Here's how the part is built. I have some questions about the finished solid (model axes, mm). A direction names the side the tool comes from. Round coordinates to 2 decimals unless told otherwise and drop trailing zeros. Write each loop counter-clockwise with the first axis right and the second up, starting at its lowest first coordinate (ties: lowest second). Pieces come first, ordered by that corner, then holes. Notation, with made-up numbers: M 23.5,78 L 72.5,78 A22 ccw 72.5,97 Z; hole C 25,58.5 d1. An arc over 180 degrees is marked long. Use a Markdown table: item, result. Add a question column.
```python
from build123d import *

# Parameters (mm, degrees)
F0_W      = 25
F0_H      = 27.7
F0_H_2    = 25
F0_W_2    = 27.7
F1_DEPTH  = 2
F0_W_3    = 1.8
F2_DEPTH  = 130
F0_H_3    = 1.8
F3_DEPTH  = 4
F4_W      = 25
F4_H      = 2
F5_DEPTH  = 80.4
F7_W      = 25
F7_H      = 2
F8_DEPTH  = 25
F6_W      = 25
F6_H      = 2
F9_DEPTH  = 25
F12_DEPTH = 25
F13_R     = 5


with BuildPart() as f1:
    # F0 (on Top) → F1 (new body)
    with BuildSketch(Plane.XY):
        with Locations((0, 26.35)):
            Rectangle(F0_W, F0_H)
        Rectangle(F0_W, F0_H_2)
        with Locations((26.35, 0)):
            Rectangle(F0_W_2, F0_H_2)
        with Locations((0, -26.35)):
            Rectangle(F0_W, F0_H)
        with Locations((-26.35, 0)):
            Rectangle(F0_W_2, F0_H_2)
    extrude(amount=F1_DEPTH)

    # F0 (on Top) → F2 (join)
    with BuildSketch(Plane.XY):
        with Locations((-41.1, 0)):
            Rectangle(F0_W_3, F0_H_2)
        with Locations((41.1, 0)):
            Rectangle(F0_W_3, F0_H_2)
    extrude(amount=F2_DEPTH)

    # F0 (on Top) → F3 (join)
    with BuildSketch(Plane.XY):
        with Locations((0, 41.1)):
            Rectangle(F0_W, F0_H_3)
        with Locations((0, -41.1)):
            Rectangle(F0_W, F0_H_3)
    extrude(amount=F3_DEPTH)

    # F4 (on face) → F5 (join)
    with BuildSketch(Plane(origin=(40.2, 0, 0), x_dir=(0, -1, 0), z_dir=(-1, 0, 0))):
        with Locations((0, 129)):
            Rectangle(F4_W, F4_H)
    extrude(amount=F5_DEPTH)

    # F7 (on face) → F8 (join)
    with BuildSketch(Plane.YZ.offset(42)):
        with Locations((0, 129)):
            Rectangle(F7_W, F7_H)
    extrude(amount=F8_DEPTH)

    # F6 (on face) → F9 (join)
    with BuildSketch(Plane(origin=(-42, 0, 0), x_dir=(0, -1, 0), z_dir=(-1, 0, 0))):
        with Locations((0, 129)):
            Rectangle(F6_W, F6_H)
    extrude(amount=F9_DEPTH)

    # F11 (on face) + F10 (on face) → F12 (cut)
    with BuildSketch(Plane(origin=(0, 0, 128), x_dir=(1, 0, 0), z_dir=(0, 0, -1))):
        with BuildLine():
            ThreePointArc((-51.5, 0), (-52.3786796564, 2.1213203436), (-54.5, 3))
            Line((-54.5, 3), (-54.5, 0))
            Line((-54.5, 0), (-51.5, 0))
        make_face()
        with BuildLine():
            Line((-54.5, 0), (-54.5, 3))
            ThreePointArc((-54.5, 3), (-56.6213203436, 2.1213203436), (-57.5, 0))
            Line((-57.5, 0), (-54.5, 0))
        make_face()
        with BuildLine():
            Line((-51.5, 0), (-54.5, 0))
            Line((-54.5, 0), (-54.5, -3))
            ThreePointArc((-54.5, -3), (-52.3786796564, -2.1213203436), (-51.5, 0))
        make_face()
        with BuildLine():
            Line((-54.5, -3), (-54.5, 0))
            Line((-54.5, 0), (-57.5, 0))
            ThreePointArc((-57.5, 0), (-56.6213203436, -2.1213203436), (-54.5, -3))
        make_face()
    with BuildSketch(Plane(origin=(0, 0, 128), x_dir=(1, 0, 0), z_dir=(0, 0, -1))):
        with BuildLine():
            Line((54.5, 0), (54.5, 3))
            ThreePointArc((54.5, 3), (52.3786796564, 2.1213203436), (51.5, 0))
            Line((51.5, 0), (54.5, 0))
        make_face()
        with BuildLine():
            ThreePointArc((57.5, 0), (56.6213203436, 2.1213203436), (54.5, 3))
            Line((54.5, 3), (54.5, 0))
            Line((54.5, 0), (57.5, 0))
        make_face()
        with BuildLine():
            Line((57.5, 0), (54.5, 0))
            Line((54.5, 0), (54.5, -3))
            ThreePointArc((54.5, -3), (56.6213203436, -2.1213203436), (57.5, 0))
        make_face()
        with BuildLine():
            Line((54.5, -3), (54.5, 0))
            Line((54.5, 0), (51.5, 0))
            ThreePointArc((51.5, 0), (52.3786796564, -2.1213203436), (54.5, -3))
        make_face()
    extrude(amount=-F12_DEPTH, mode=Mode.SUBTRACT)

    # F13
    f13_edges = [f1.edges().sort_by_distance(p)[0] for p in [
        (67, 12.5, 129),
        (67, -12.5, 129),
        (-67, 12.5, 129),
        (-67, -12.5, 129),
    ]]
    fillet(f13_edges, radius=F13_R)


solid = f1.part
```
Item 1: Imagine slicing it at B-B on z = 120. List the corners of the cut face in (x, y) for me, plus the area to 3 significant figures.
Item 2: Imagine slicing it at D-D on x = -20. List the corners of the cut face in (y, z) for me, plus the area to 3 significant figures.
Item 3: Imagine slicing it at A-A on x = -6. List the corners of the cut face in (y, z) for me.
Item 4: For pin 1 Ø7.5 at (x, y) = (56.5, -5.5) entering from -Z; pin 2 Ø1.2 at (y, z) = (31.5, 2) entering from -X; pin 3 Ø8 at (x, z) = (-38.5, 33.5) entering from -Y, each with a flat end and sliding along its axis, tell me the tip position at first contact or that it passes through.
Item 5: On a 3-axis mill with a long thin cutter (end or side, diameter ignored), from which of +Z, -Z, +X, -X, +Y, -Y can I reach the whole of each face in a straight line? I mean faces 5 (the face through (-12.5, -27, 1)), 6 (the face through (12.5, 27, 1)), 7 (the face through (-12.5, 27, 1)), 8 (the face through (42, 0, 63)). Say none if no direction works.
Item 6: If we mould it in two halves opening along Z, with no side actions, what happens to faces 1 (the face through (-1, 1, 0)), 2 (the face through (-1, 1, 2)), 3 (the face through (-65.5, 11.07, 129.01)), 4 (the face through (40.2, 0, 64))? For each: +Z half, -Z half, draft (parallel to the pull), parting line (faces both ways), or undercut.
Item 7: I need wall thicknesses on probe 1 along X at (y, z) = (-10, 121.5); probe 2 along Z at (x, y) = (-20, 9.5); probe 3 along Z at (x, y) = (-11.5, -14). Which ranges of each line are inside material? Lowest first, please. Write a range as from..to.
Item 8: Imagine slicing it at C-C on y = -5. List the corners of the cut face in (x, z) for me.
The answers:
| question | item | result |
|---|---|---|
| 1 | outline | M -42,-12.5 L -40.2,-12.5 L -40.2,12.5 L -42,12.5 Z; M 40.2,-12.5 L 42,-12.5 L 42,12.5 L 40.2,12.5 Z |
| 1 | area | 90.0 mm² |
| 2 | outline | M -12.5,0 L 12.5,0 L 12.5,2 L -12.5,2 Z; M -12.5,128 L 12.5,128 L 12.5,130 L -12.5,130 Z |
| 2 | area | 100 mm² |
| 3 | outline | M -42,0 L 42,0 L 42,4 L 40.2,4 L 40.2,2 L -40.2,2 L -40.2,4 L -42,4 Z; M -12.5,128 L 12.5,128 L 12.5,130 L -12.5,130 Z |
| 4 | pin 1 | z = 128 |
| 4 | pin 2 | x = -12.5 |
| 4 | pin 3 | y = -12.5 |
| 5 | face 5 | +Z, -Z, -X, -Y |
| 5 | face 6 | +Z, -Z, +X, +Y |
| 5 | face 7 | +Z, -Z, -X, +Y |
| 5 | face 8 | -Z, +X, +Y, -Y |
| 6 | face 1 | -Z half |
| 6 | face 2 | undercut |
| 6 | face 3 | draft |
| 6 | face 4 | undercut |
| 7 | probe 1 | -42..-40.2, 40.2..42 |
| 7 | probe 2 | 0..2, 128..130 |
| 7 | probe 3 | 0..2 |
| 8 | outline | M -67,128 L -42,128 L -42,0 L 42,0 L 42,128 L 67,128 L 67,130 L -67,130 Z; hole M -40.2,2 L 40.2,2 L 40.2,128 L -40.2,128 Z |
